```python
from build123d import *

# Parameters (mm, degrees)
FILLET1_R = 4
FILLET2_R = 10


with BuildPart() as part:
    # Sketch1 → Revolve1 (revolve)
    with BuildSketch(Plane.XY, mode=Mode.PRIVATE) as revolve1_sk:
        Polygon((0, 0), (-100, 0), (-100, 6), (-15, 13.4365364), (-15, 30), (-10, 30), (-10, 1500), (0, 1500), align=None)
    revolve(revolve1_sk.sketch.rotate(Axis((0, 0, 0), (0, -1, 0)), 270), axis=Axis((0, 0, 0), (0, -1, 0)))

    # Fillet1
    fillet1_edges = [part.edges().sort_by_distance(p)[0] for p in [
        (0, 6, -100),
    ]]
    fillet(fillet1_edges, radius=FILLET1_R)

    # Fillet2
    fillet2_edges = [part.edges().sort_by_distance(p)[0] for p in [
        (0, 13.4365364, -15),
    ]]
    fillet(fillet2_edges, radius=FILLET2_R)


solid = part.part
```
Can you work these out from the model? Positions are in its coordinate system, mm. A direction names the side the tool comes from. Coordinates: 2 decimals unless noted, no trailing zeros. Loops run counter-clockwise (first coordinate to the right, second up) from the corner with the lowest first, then second, coordinate; pieces in that order, holes last. Notation, with made-up numbers: (47.25, 23) - (100.25, 23) arc R20 cw to (100.25, 56) - close; hole circle Ø9 at (38, -6). An arc over 180 degrees is marked (long way). Use a Markdown table: item, result.
Item 1: I want a section at A-A on y = 399.5. Please give me the cut outline in (x, z), and give its area (3 significant figures).
Numbers:
| item | result |
|---|---|
| outline | circle Ø20 at (0, 0) |
| area | 314 mm2 |
Item 2: For faces 1 (the face through (-30.04, 1.18, 95.38)), 2 (the face through (-0.66, 26.352, -14.985)), which set-ups out of +Z, -Z, +X, -X, +Y, -Y let a thin tool reach every point of the face, with its end or its side?
Numbers:
| item | result |
|---|---|
| face 1 | +Y, -Y |
| face 2 | +Y |
Item 3: Will this pin go through, and if not, where does the flat tip stop? pin 1 (1 mm diameter, centred on y = 1037, z = -9, fed in from -X).
Numbers:
| item | result |
|---|---|
| pin 1 | stops at x = -5.27 |
Item 4: We'd pull the mould along Y, two halves only. Please class faces 3 (the face through (3, 30, 10)), 4 (the face through (-1, 0, 1)): released by +Y, released by -Y, zero draft, split by the parting line, or undercut.
Numbers:
| item | result |
|---|---|
| face 3 | released by +Y |
| face 4 | released by -Y |
Item 5: If I drill on probe 1 along Y at (x, z) = (68.5, 5.5); probe 2 along Y at (x, z) = (17.5, -31.5), over which ranges is the centre line in solid material (lowest first)? Write a range as from..to.
Numbers:
| item | result |
|---|---|
| probe 1 | y = 0..8.74 |
| probe 2 | y = 0..11.6 |
